Autodesk Inventor part; units mm, degrees
ref_plane "YZ Plane" through (0, 0, 0) normal (1, 0, 0) x (0, 1, 0)
ref_plane "XZ Plane" through (0, 0, 0) normal (0, 1, 0) x (-1, 0, 0)
ref_plane "XY Plane" through (0, 0, 0) normal (0, 0, 1) x (1, 0, 0)
sketch "Эскиз1" plane through (0, 0, 0) normal (0, 1, 0) x (-1, 0, 0)
  line L0 (-40, 6.35) -> (40, 6.35)
  line L1 (40, 6.35) -> (40, -6.35)
  line L2 (40, -6.35) -> (-40, -6.35)
  line L3 (-40, -6.35) -> (-40, 6.35)
  line L4 (-40, 6.35) -> (40, -6.35) construction
  line L5 (40, 6.35) -> (-40, -6.35) construction
  point P0 (0, 0)
  dimension "d0" = 80
  dimension "d1" = 12.7
extrude "Выдавливание1" add sketch "Эскиз1" along normal blind 12.7
sketch "Эскиз2" plane through (0, 12.7, 0) normal (0, 1, 0) x (1, 0, 0)
  point P0 (0, 0)
  point P1 (-35, 0)
  point P2 (-20, 0)
  point P3 (20, 0)
  point P4 (35, 0)
  dimension "d4" = 15
  dimension "d5" = 40
  dimension "d6" = 15
  dimension "d7" = 20
hole "Отверстие1" at (-35, 12.7, 0) at (-20, 12.7, 0) direction (0, -1, 0) diameter 3.242 end through all
hole "Отверстие2" at (20, 12.7, 0) at (35, 12.7, 0) direction (0, -1, 0) diameter 4.134 end through all
sketch "Эскиз3" plane through (-40, 0, 6.35) normal (0, 0, 1) x (1, 0, 0)
  line L0 (80, 0) -> (0, 0)
  arc A0 (40, 11.249) -> (40, 1.451) centre (37.5, 6.35) ccw
  arc A1 (40, 1.451) -> (40, 11.249) centre (42.5, 6.35) ccw
  line L1 (80, 0) -> (80, 12.7)
  point P0 (40, 0)
  point P1 (40, 0)
  point P2 (80, 6.35)
  dimension "d22" = 11
  dimension "d23" = 11
  dimension "d24" = 5
extrude "Выдавливание2" cut sketch "Эскиз3" against normal through all
sketch "Эскиз4" plane through (0, 12.7, 0) normal (0, 1, 0) x (1, 0, 0)
  line L0 (40, 6.35) -> (-40, 6.35)
  line L1 (-8.5, -6.35) -> (8.5, -6.35)
  line L2 (8.5, -6.35) -> (8.5, 6.35)
  line L3 (8.5, 6.35) -> (-8.5, 6.35)
  line L4 (-8.5, 6.35) -> (-8.5, -6.35)
  line L5 (-8.5, -6.35) -> (8.5, 6.35) construction
  line L6 (8.5, -6.35) -> (-8.5, 6.35) construction
  point P0 (0, 0)
  dimension "d27" = 17
extrude "Выдавливание3" add sketch "Эскиз4" along normal blind 1 draft -50
fillet "Сопряжение1" radius 5 4 edges at (7.3082, 13.7, 0) (0, 13.7, 5.1582) (-7.3082, 13.7, 0) (0, 13.7, -5.1582)
sketch "Эскиз5" plane through (0, 0, 0) normal (0, -1, 0) x (1, 0, 0)
  line L0 (40, 6.35) -> (-40, 6.35)
  line L1 (-8.5, -6.35) -> (8.5, -6.35)
  line L2 (8.5, -6.35) -> (8.5, 6.35)
  line L3 (8.5, 6.35) -> (-8.5, 6.35)
  line L4 (-8.5, 6.35) -> (-8.5, -6.35)
  line L5 (-8.5, -6.35) -> (8.5, 6.35) construction
  line L6 (8.5, -6.35) -> (-8.5, 6.35) construction
  point P0 (0, 0)
  dimension "d31" = 17
extrude "Выдавливание4" add sketch "Эскиз5" along normal blind 1 draft -50
fillet "Сопряжение2" radius 5 4 edges at (-7.3082, -1, 0) (0, -1, 5.1582) (7.3082, -1, 0) (0, -1, -5.1582)
chamfer "Фаска1" distance 0.5 angle 45 8 edges at (-35, 12.7, -1.621) (-20, 12.7, -1.621) (20, 12.7, -2.067) (35, 12.7, -2.067) (20, 0, -2.067) (35, 0, -2.067) (-20, 0, -1.621) (-35, 0, -1.621)
properties part number "Weight Sensor" material "Алюминий 6061-AHC"
The model under review builds one solid part; all positions refer to its coordinate system, in mm. A direction names the side the tool comes from. Round coordinates to 2 decimals unless told otherwise and drop trailing zeros. Loops run counter-clockwise (first coordinate to the right, second up) from the corner with the lowest first, then second, coordinate; pieces in that order, holes last. Notation, with made-up numbers: M 48.25,20 L 95.25,20 A28 cw 95.25,40 Z; hole C 82,-36 d1. An arc over 180 degrees is marked long. Answer as a JSON object with one key per item and string values.
Item 1: We need section B-B, the plane x = 2.5. State the section outline as (y, z) points, and give its area (3 significant figures).
Check sheet entries:
{"outline": "M -1,-3.34 A5 ccw 0.01,-6.35 L 0.85,-6.35 L 0.85,6.35 L 0.01,6.35 A5 ccw -1,3.34 Z; M 11.85,-6.35 L 12.69,-6.35 A5 ccw 13.7,-3.34 L 13.7,3.34 A5 ccw 12.69,6.35 L 11.85,6.35 Z", "area": "43.1 mm2"}
Item 2: Clearance check with flat-ended pins moving along their axes: P1, Ø3, axis at x = -35, z = 0, coming from the -Y side; P2, Ø5.5, axis at x = 35, z = 0, coming from the +Y side; P3, Ø5, axis at x = -20, z = 0, coming from the -Y side. State where each tip first meets the part, or that it passes through.
Check sheet entries:
{"P1": "through", "P2": "y = 12.7", "P3": "y = 0"}
Item 3: We need section D-D, the plane z = 4.25. State the section outline as (x, y) points, and give its area (3 significant figures).
Check sheet entries:
{"outline": "M -40,0 L -8.49,0 A5 ccw -6.4,-0.92 L 6.4,-0.92 A5 ccw 8.49,0 L 40,0 L 40,12.7 L 8.49,12.7 A5 ccw 6.4,13.62 L -6.4,13.62 A5 ccw -8.49,12.7 L -40,12.7 Z; hole M 0,1.45 A5.5 ccw long 0,11.25 A5.5 ccw long Z", "area": "896 mm2"}
Item 4: For line 1 along Z through (x, y) = (-35, 5.5); line 2 along X through (y, z) = (8.75, 0); line 3 along X through (y, z) = (4, 0), list the stretches that pass through material, from the lowest coordinate up.
Check sheet entries:
{"line 1": "-6.35 to -1.62, 1.62 to 6.35", "line 2": "-40 to -36.62, -33.38 to -21.62, -18.38 to -7.45, 7.45 to 17.93, 22.07 to 32.93, 37.07 to 40", "line 3": "-40 to -36.62, -33.38 to -21.62, -18.38 to -7.47, 7.47 to 17.93, 22.07 to 32.93, 37.07 to 40"}
Item 5: The part is to be moulded in two halves that separate along Z. For faces 1 (the face through (37.018, 6.268, -0.448)), 2 (the face through (0.166, 13.434, -4.948)), 3 (the face through (7.998, 6.193, 0.089)), say which applies: +Z half, -Z half, draft (parallel to the pull), parting line (faces both ways), or undercut.
Check sheet entries:
{"face 1": "undercut", "face 2": "-Z half", "face 3": "draft"}
Item 6: Tool access review of faces 4 (the face through (-24, 12.7, 0)), 5 (the face through (24, 0, 0)), 6 (the face through (-7.998, 6.507, 0.089)), 7 (the face through (24, 12.7, 0)): name each direction out of +Z, -Z, +X, -X, +Y, -Y from which nothing blocks a thin tool from reaching the whole face with its end or side.
Check sheet entries:
{"face 4": "+Z, -Z, -X, +Y", "face 5": "+Z, -Z, +X, -Y", "face 6": "+Z, -Z", "face 7": "+Z, -Z, +X, +Y"}
Item 7: We need section A-A, the plane y = 6.35. State the section outline as (x, z) points.
Check sheet entries:
{"outline": "M -40,-6.35 L -8,-6.35 L -8,6.35 L -40,6.35 Z; M 8,-6.35 L 40,-6.35 L 40,6.35 L 8,6.35 Z; hole C -35,0 d3.24; hole C -20,0 d3.24; hole C 20,0 d4.13; hole C 35,0 d4.13"}
Item 8: We need section C-C, the plane x = 35. State the section outline as (y, z) points, and give its area (3 significant figures).
Check sheet entries:
{"outline": "M 0,-6.35 L 12.7,-6.35 L 12.7,-2.57 L 12.2,-2.07 L 0.5,-2.07 L 0,-2.57 Z; M 0,2.57 L 0.5,2.07 L 12.2,2.07 L 12.7,2.57 L 12.7,6.35 L 0,6.35 Z", "area": "108 mm2"}
